Source: CAD feature listing. Evaluate the final solid. Frame: model axes, mm. Face numbers are marked on the shaded views. A direction names the side the tool comes from. Give positions to 0.01 mm unless a question says otherwise; leave off trailing zeros. Loops run counter-clockwise (first coordinate to the right, second up) from the corner with the lowest first, then second, coordinate; pieces in that order, holes last. Notation, with made-up numbers: M -32,20 L 20,20 A20 cw 20,35 Z; hole C -36.5,84.25 d8. An arc over 180 degrees is marked long. Answer in a Markdown table with one row per item.
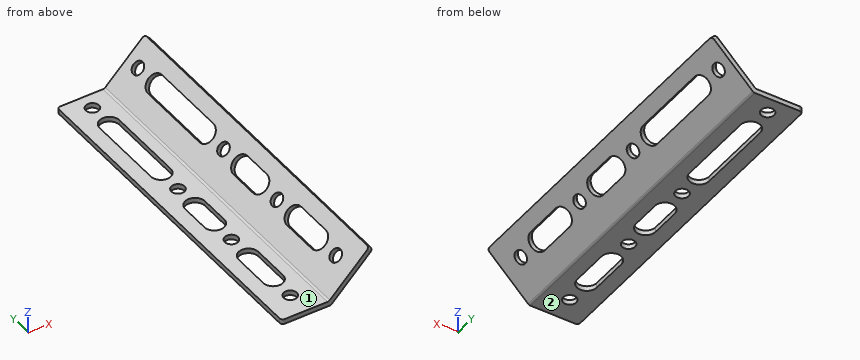
```python
from build123d import *

# Parameters (mm, degrees)
EXTRUDE_1_DEPTH     = 105
SKETCH_2_R          = 2
CUT_EXTRUDE_1_DEPTH = 107.775508677
SKETCH_3_R          = 2
CUT_EXTRUDE_2_DEPTH = 110.207453302
FILLET_1_R          = 1


with BuildPart() as part:
    # 草图1 → 拉伸-薄壁1 (new body)
    with BuildSketch(Plane(origin=(0, 0, 0), x_dir=(1, 0, 0), z_dir=(0, 1, 0))):
        Polygon((-15, 0), (0, 0), (12.727922061, -12.727922061), (11.66726189, -13.788582233), (-0.621320344, -1.5), (-15, -1.5), align=None)
    extrude(amount=EXTRUDE_1_DEPTH)

    # 草图2 → 切除-拉伸1 (cut, through all)
    with BuildSketch(Plane.XY.offset(1.5)):
        with Locations((-7.5, 100)):
            Circle(SKETCH_2_R)
        with Locations((-7.5, 60)):
            Circle(SKETCH_2_R)
        with Locations((-7.5, 35)):
            Circle(SKETCH_2_R)
        with Locations((-7.5, 7.5)):
            Circle(SKETCH_2_R)
        with BuildLine():
            Line((-4.5, 92), (-4.5, 68))
            ThreePointArc((-4.5, 68), (-7.5, 65), (-10.5, 68))
            Line((-10.5, 68), (-10.5, 92))
            ThreePointArc((-10.5, 92), (-7.5, 95), (-4.5, 92))
        make_face()
        with BuildLine():
            Line((-4.5, 52), (-4.5, 43))
            ThreePointArc((-4.5, 43), (-7.5, 40), (-10.5, 43))
            Line((-10.5, 43), (-10.5, 52))
            ThreePointArc((-10.5, 52), (-7.5, 55), (-4.5, 52))
        make_face()
        with BuildLine():
            Line((-4.5, 27), (-4.5, 15.5))
            ThreePointArc((-4.5, 15.5), (-7.5, 12.5), (-10.5, 15.5))
            Line((-10.5, 15.5), (-10.5, 27))
            ThreePointArc((-10.5, 27), (-7.5, 30), (-4.5, 27))
        make_face()
    extrude(amount=-CUT_EXTRUDE_1_DEPTH, mode=Mode.SUBTRACT)

    # 草图3 → 切除-拉伸2 (cut, through all)
    with BuildSketch(Plane(origin=(11.66726189, 0, 13.788582233), x_dir=(0.7071067811865562, 0, 0.7071067811865389), z_dir=(-0.7071067811865389, 0, 0.7071067811865562))):
        with BuildLine():
            Line((-4.5, 68), (-4.5, 92))
            ThreePointArc((-4.5, 92), (-7.5, 95), (-10.5, 92))
            Line((-10.5, 92), (-10.5, 68))
            ThreePointArc((-10.5, 68), (-7.5, 65), (-4.5, 68))
        make_face()
        with BuildLine():
            Line((-4.5, 43), (-4.5, 52))
            ThreePointArc((-4.5, 52), (-7.5, 55), (-10.5, 52))
            Line((-10.5, 52), (-10.5, 43))
            ThreePointArc((-10.5, 43), (-7.5, 40), (-4.5, 43))
        make_face()
        with BuildLine():
            Line((-4.5, 15.5), (-4.5, 27))
            ThreePointArc((-4.5, 27), (-7.5, 30), (-10.5, 27))
            Line((-10.5, 27), (-10.5, 15.5))
            ThreePointArc((-10.5, 15.5), (-7.5, 12.5), (-4.5, 15.5))
        make_face()
        with Locations((-7.5, 100)):
            Circle(SKETCH_3_R)
        with Locations((-7.5, 60)):
            Circle(SKETCH_3_R)
        with Locations((-7.5, 35)):
            Circle(SKETCH_3_R)
        with Locations((-7.5, 7.5)):
            Circle(SKETCH_3_R)
    extrude(amount=-CUT_EXTRUDE_2_DEPTH, mode=Mode.SUBTRACT)

    # 圆角1
    fillet_1_edges = [part.edges().sort_by_distance(p)[0] for p in [
        (-15, 105, 0.75),
        (-15, 0, 0.75),
        (12.197591975, 0, 13.258252147),
        (12.197591975, 105, 13.258252147),
        (-0.621320344, 52.5, 1.5),
        (0, 52.5, 0),
    ]]
    fillet(fillet_1_edges, radius=FILLET_1_R)


solid = part.part
```
Q1. Contact query for flat-ended pins moving along their axis: pin 1 Ø3 at (x, y) = (-7.5, 35) entering from +Z; pin 2 Ø1.6 at (y, z) = (49, 1) entering from +X; pin 3 Ø4 at (x, y) = (-1.5, 60.5) entering from +Z; pin 4 Ø1 at (y, z) = (49, 4.5) entering from -X. Output: stop coordinate, or through.
Values follow:
| item | result |
|---|---|
| pin 1 | through |
| pin 2 | x = 1.8 |
| pin 3 | z = 2.62 |
| pin 4 | x = 1.88 |
Q2. Section query A-A (y = 25.5). Output: boundary loops of the cut face in (x, z), plus the area to 3 significant figures.
Values follow:
| item | result |
|---|---|
| outline | M -15,0 L -10.5,0 L -10.5,1.5 L -15,1.5 Z; M -4.5,0 L -0.41,0 A1 ccw 0.29,0.29 L 5.3,5.3 L 4.24,6.36 L -0.33,1.79 A1 cw -1.04,1.5 L -4.5,1.5 Z; M 8.49,10.61 L 9.55,9.55 L 12.73,12.73 L 11.67,13.79 Z |
| area | 30.6 mm^2 |
Q3. Section query B-B (x = -7.5). Give the number of separate pieces and of enclosed holes in the cut face, plus the area to 4 significant figures.
Values follow:
| item | result |
|---|---|
| separate pieces | 8 |
| enclosed holes | 0 |
| area | 39.75 mm^2 |
Q4. Section query D-D (x = -12). Output: boundary loops of the cut face in (y, z).
Values follow:
| item | result |
|---|---|
| outline | M 0,0 L 105,0 L 105,1.5 L 0,1.5 Z |
Q5. Ray query, probe 1 along Z at (x, y) = (-4.5, 56.5); probe 2 along Z at (x, y) = (4.75, 55); probe 3 along X at (y, z) = (24, 13). Return the intervals inside material, ascending. Write a range as from..to.
Values follow:
| item | result |
|---|---|
| probe 1 | 0..1.5 |
| probe 2 | 4.75..6.87 |
| probe 3 | 10.88..12.46 |
Q6. Reachability of the marked faces 1 and 2 from +Z, -Z, +X, -X, +Y, -Y: full face, straight path, thin tool, end or side. Return the list, or none.
Values follow:
| item | result |
|---|---|
| face 1 | +Z, -X, +Y, -Y |
| face 2 | -Z, +X, -X, +Y, -Y |
Q7. Section query C-C (y = 100). Output: boundary loops of the cut face in (x, z), plus the area to 3 significant figures.
Values follow:
| item | result |
|---|---|
| outline | M -15,0 L -9.5,0 L -9.5,1.5 L -15,1.5 Z; M -5.5,0 L -0.41,0 A1 ccw 0.29,0.29 L 6.01,6.01 L 4.95,7.07 L -0.33,1.79 A1 cw -1.04,1.5 L -5.5,1.5 Z; M 7.78,9.9 L 8.84,8.84 L 12.73,12.73 L 11.67,13.79 Z |
| area | 36.6 mm^2 |
